For this review, use the dimensioned drawing (mm, ordinates from the lowest corner) and the shaded views. A direction names the side the tool comes from. Round coordinates to 2 decimals unless told otherwise and drop trailing zeros. Order: outer loops, then holes, each group sorted by start corner. A loop starts at its lowest first (then second) coordinate and runs counter-clockwise, first axis right, second up. Notation, with made-up numbers: M 25,71.25 L 34,71.25 A18 cw 34,78.25 Z; hole C 70,48 d9. An arc over 180 degrees is marked long. One line per item, written item: value. Start each with the question number.
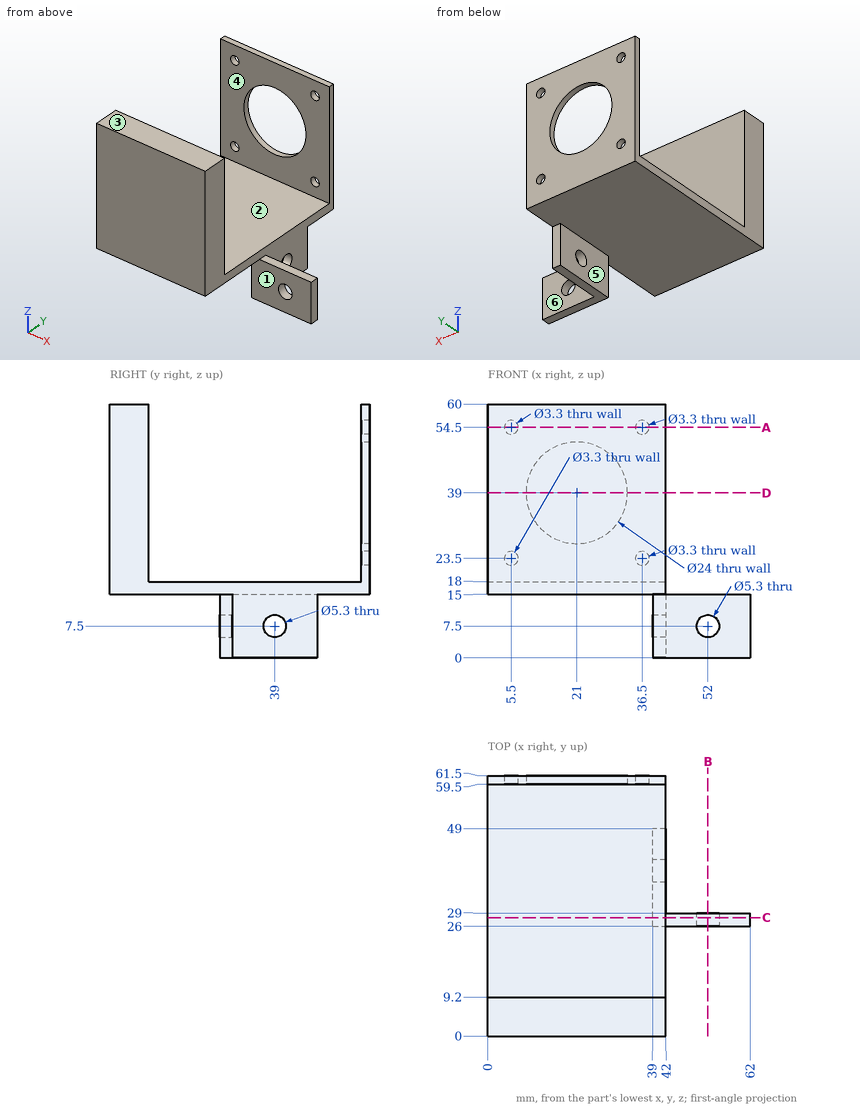
Item 1: Clearance check with flat-ended pins moving along their axes: P1, Ø21, axis at x = 17, y = 30.5, coming from the +Z side; P2, Ø10, axis at y = 29.5, z = 7, coming from the -X side; P3, Ø3, axis at x = 5.5, z = 23.5, coming from the +Y side. State where each tip first meets the part, or that it passes through.
Item 2: Consider section D-D, the plane z = 39. Give the boundary of the cut face in (x, y).
Item 3: Consider section C-C, the plane y = 28. Give the boundary of the cut face in (x, z).
Item 4: Consider section A-A, the plane z = 54.5. Give the boundary of the cut face in (x, y).
Item 5: The part is to be moulded in two halves that separate along Y. For the marked faces 1, 2 and 3, say which applies: pulls with the +Y half, pulls with the -Y half, needs draft (parallel to the pull), parting line crosses it, or undercut.
Item 6: Consider section B-B, the plane x = 52. Give the boundary of the cut face in (y, z).
Item 7: Wall thickness on L1, parallel to Z at x = 5.5, y = 61.05; L2, parallel to Y at x = 7, z = 27; L3, parallel to X at y = 60, z = 54: over which ranges is each line inside the solid? List them lowest first.
Item 8: Machinability: for the marked faces 4, 5 and 6, which of the approach directions +Z, -Z, +X, -X, +Y, -Y give a long, thin tool a straight path to every point of the face, cutting with its end or side? Answer none if there is none.
Computed:
1. P1: stops at z = 18
1. P2: stops at x = 39
1. P3: stops at y = 9.2
2. outline: M 0,0 L 42,0 L 42,9.2 L 0,9.2 Z; M 0,59.5 L 9,59.5 L 9,61.5 L 0,61.5 Z; M 33,59.5 L 42,59.5 L 42,61.5 L 33,61.5 Z
3. outline: M 0,15 L 39,15 L 39,0 L 62,0 L 62,15 L 42,15 L 42,18 L 0,18 Z; hole C 52,7.5 d5.3
4. outline: M 0,0 L 42,0 L 42,9.2 L 0,9.2 Z; M 0,59.5 L 3.85,59.5 L 3.85,61.5 L 0,61.5 Z; M 7.15,59.5 L 34.85,59.5 L 34.85,61.5 L 7.15,61.5 Z; M 38.15,59.5 L 42,59.5 L 42,61.5 L 38.15,61.5 Z
5. face 1: pulls with the -Y half
5. face 2: undercut
5. face 3: needs draft
6. outline: M 26,0 L 29,0 L 29,4.85 L 26,4.85 Z; M 26,10.15 L 29,10.15 L 29,15 L 26,15 Z
7. L1: z = 15 to 21.85, 25.15 to 52.85, 56.15 to 60
7. L2: y = 0 to 9.2, 59.5 to 61.5
7. L3: x = 0 to 3.93, 7.07 to 34.93, 38.07 to 42
8. face 4: +Z, +X, -X
8. face 5: -Z, -X, +Y, -Y
8. face 6: +Z, -Z, +X, +Y
